Drawing for the job (mm, zero at the part's lowest x, y, z). Give positions to 0.01 mm unless a question says otherwise; leave off trailing zeros. Order: outer loops, then holes, each group sorted by start corner. A loop starts at its lowest first (then second) coordinate and runs counter-clockwise, first axis right, second up. Notation, with made-up numbers: (67.5, -10.5) -> (122.5, -10.5) arc R21 cw to (122.5, 20.5) -> close; hole circle Ø2 at (53, 44). An arc over 180 degrees is marked (long way). One line per item, written item: value. Start each with the question number.
(1) Probe line 1 (Y direction, x = 2.05, z = 34) (1 decimal); line 2 (Y direction, x = 0.9, z = 32.5); line 3 (Z direction, x = 3.55, y = 42). List the from-to ranges inside material, lowest first.
(2) Pin check, flat tips, straight feed: pin 1 (2 mm diameter, centred on x = 1.5, z = 23, fed in from +Y); pin 2 (2 mm diameter, centred on x = 1, z = 30, fed in from -Y). Stop position of each tip, or through.
(3) Saw through at D-D on z = 15. Give the cut face in (x, y).
(4) Saw through at C-C on y = 44. Give the cut face in (x, z).
(5) Saw through at B-B on z = 25. Give the cut face in (x, y).
(6) Saw through at A-A on x = 0.9. Give the cut face in (y, z) (1 decimal), plus the area to 3 significant figures.
(7) Two-plate mould, pull along Z, no slides. Class the marked faces 1, 2, 3 and 4: +Z half, -Z half, draft (parallel to the pull), parting line (faces both ways), or undercut.
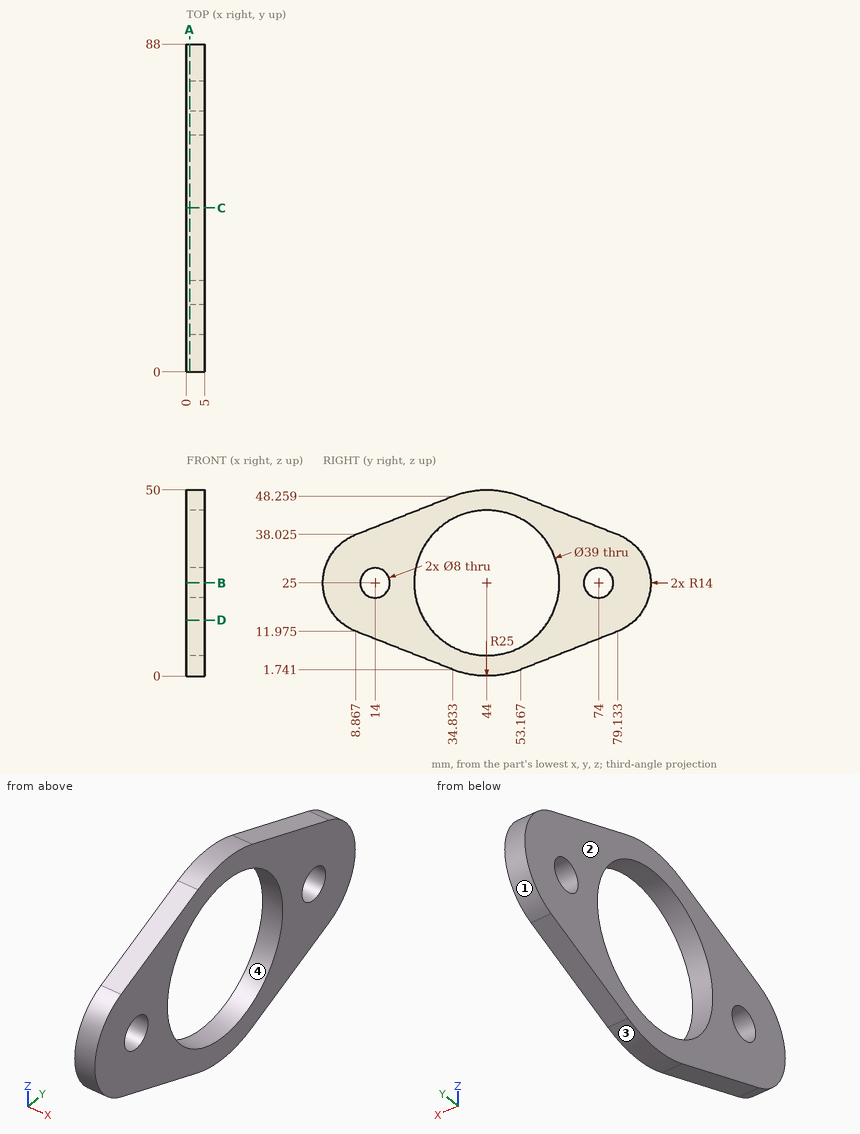
Results below:
1. line 1: y = 3.3 to 26.7, 61.3 to 84.7
1. line 2: y = 2.18 to 26, 62 to 85.82
1. line 3: z = 0.08 to 5.6, 44.4 to 49.92
2. pin 1: stops at y = 87.96
2. pin 2: stops at y = 0.58
3. outline: (0, 4.2) -> (5, 4.2) -> (5, 27.26) -> (0, 27.26) -> close; (0, 60.74) -> (5, 60.74) -> (5, 83.8) -> (0, 83.8) -> close
4. outline: (0, 0) -> (5, 0) -> (5, 5.5) -> (0, 5.5) -> close; (0, 44.5) -> (5, 44.5) -> (5, 50) -> (0, 50) -> close
5. outline: (0, 0) -> (5, 0) -> (5, 10) -> (0, 10) -> close; (0, 18) -> (5, 18) -> (5, 24.5) -> (0, 24.5) -> close; (0, 63.5) -> (5, 63.5) -> (5, 70) -> (0, 70) -> close; (0, 78) -> (5, 78) -> (5, 88) -> (0, 88) -> close
6. outline: (8.9, 12) -> (34.8, 1.7) arc R25 ccw to (53.2, 1.7) -> (79.1, 12) arc R14 ccw to (79.1, 38) -> (53.2, 48.3) arc R25 ccw to (34.8, 48.3) -> (8.9, 38) arc R14 ccw to start; hole circle Ø8 at (14, 25); hole circle Ø39 at (44, 25); hole circle Ø8 at (74, 25)
6. area: 1,820 mm²
7. face 1: parting line
7. face 2: draft
7. face 3: -Z half
7. face 4: undercut
